Here's the drawing with two shaded views (mm, measured from the low corner). I have some questions. Coordinates: 2 decimals unless noted, no trailing zeros. Order: outer loops, then holes, each group sorted by start corner. A loop starts at its lowest first (then second) coordinate and runs counter-clockwise, first axis right, second up. Notation, with made-up numbers: (-17, -31.5) -> (24, -31.5) arc R26 cw to (24, -2.5) -> close; hole circle Ø7 at (25, -16.5). An arc over 180 degrees is marked (long way). Return JSON: item names as keys, results as strings. Group by question number.
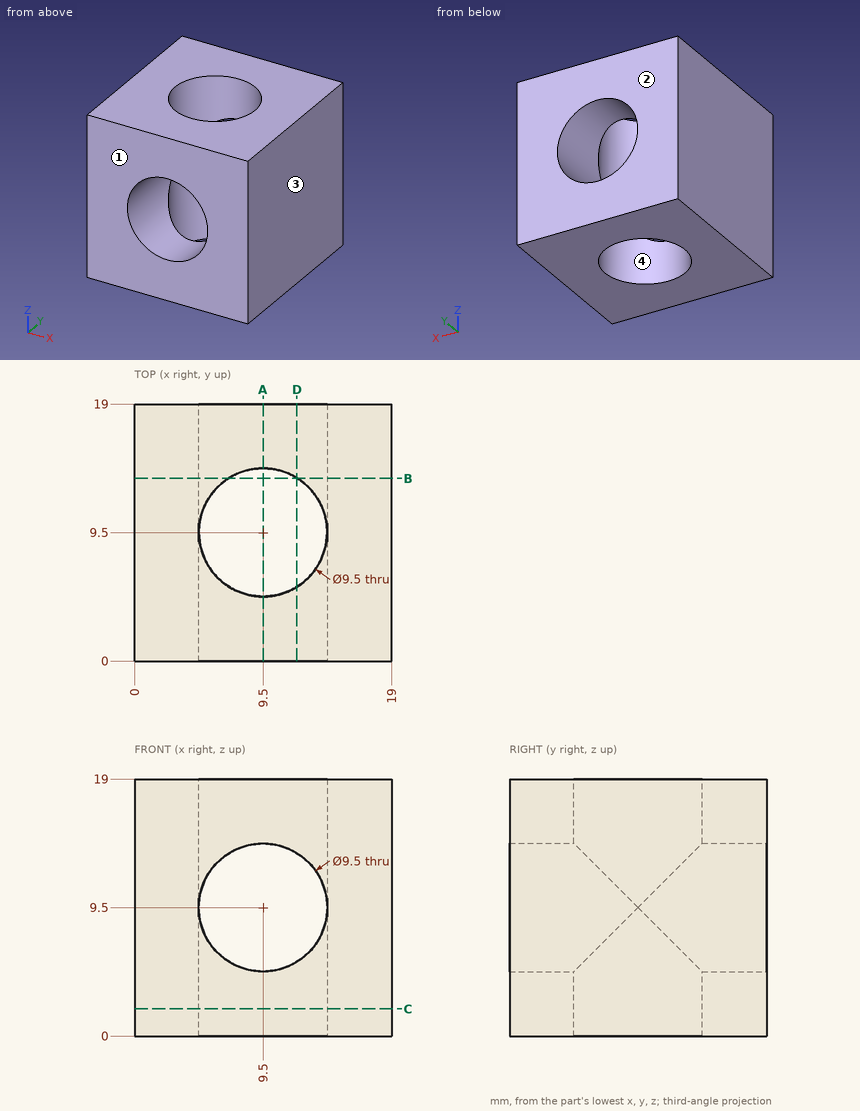
Q1. I want a section at D-D on x = 12. Please give me the cut outline in (y, z).
Q2. I need wall thicknesses on line 1 along X through (y, z) = (9.75, 5); line 2 along Z through (x, y) = (13.5, 15). Which ranges of each line are inside material? Lowest first, please. Write a range as from..to.
Q3. I want a section at B-B on y = 13.5. Please give me the cut outline in (x, z), and give its area (3 significant figures).
Q4. I want a section at A-A on x = 9.5. Please give me the cut outline in (y, z).
Q5. I want a section at C-C on z = 2. Please give me the cut outline in (x, y).
Q6. We'd pull the mould along Y, two halves only. Please class the marked faces 1, 2, 3 and 4: pulls with the +Y half, pulls with the -Y half, needs draft (parallel to the pull), parting line crosses it, or undercut.
Response values:
{
 "1": {"outline": "(0, 0) -> (5.46, 0) -> (5.46, 5.46) -> (0, 5.46) -> close; (0, 13.54) -> (5.46, 13.54) -> (5.46, 19) -> (0, 19) -> close; (13.54, 0) -> (19, 0) -> (19, 5.46) -> (13.54, 5.46) -> close; (13.54, 13.54) -> (19, 13.54) -> (19, 19) -> (13.54, 19) -> close"},
 "2": {"line 1": "x = 0..4.76, 14.24..19", "line 2": "z = 0..6.94, 12.06..19"},
 "3": {"outline": "(0, 0) -> (6.94, 0) -> (6.94, 5.5) arc R4.75 cw to (6.94, 13.5) -> (6.94, 19) -> (0, 19) -> close; (12.06, 0) -> (19, 0) -> (19, 19) -> (12.06, 19) -> (12.06, 13.5) arc R4.75 cw to (12.06, 5.5) -> close", "area": "239 mm²"},
 "4": {"outline": "(0, 0) -> (4.75, 0) -> (4.75, 4.75) -> (0, 4.75) -> close; (0, 14.25) -> (4.75, 14.25) -> (4.75, 19) -> (0, 19) -> close; (14.25, 0) -> (19, 0) -> (19, 4.75) -> (14.25, 4.75) -> close; (14.25, 14.25) -> (19, 14.25) -> (19, 19) -> (14.25, 19) -> close"},
 "5": {"outline": "(0, 0) -> (19, 0) -> (19, 19) -> (0, 19) -> close; hole circle Ø9.5 at (9.5, 9.5)"},
 "6": {"face 1": "pulls with the -Y half", "face 2": "pulls with the +Y half", "face 3": "needs draft", "face 4": "undercut"}
}
